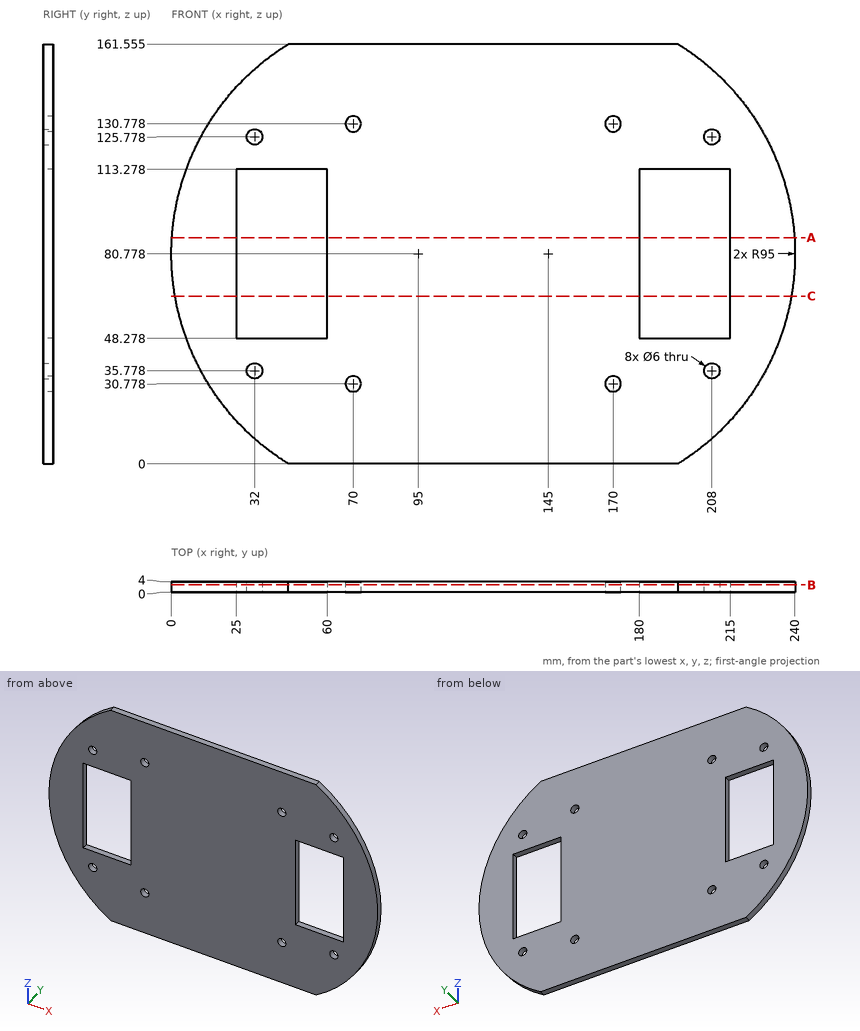
The drawing under review shows one solid part. Ordinate dimensions are in mm from its lowest x, y, z. Round coordinates to 2 decimals unless told otherwise and drop trailing zeros. Order: outer loops, then holes, each group sorted by start corner. A loop starts at its lowest first (then second) coordinate and runs counter-clockwise, first axis right, second up. Notation, with made-up numbers: (67, 20.5) -> (76, 20.5) arc R6 cw to (76, 24.5) -> close; hole circle Ø10 at (-1.75, -15.75). An arc over 180 degrees is marked (long way). Use a Markdown table: item, result.
Q1. We need section C-C on z = 64.5. Write out the cut boundary in (x, y) (1 decimal).
Values:
| item | result |
|---|---|
| outline | (1.4, 0) -> (25, 0) -> (25, 4) -> (1.4, 4) -> close; (60, 0) -> (180, 0) -> (180, 4) -> (60, 4) -> close; (215, 0) -> (238.6, 0) -> (238.6, 4) -> (215, 4) -> close |
Q2. Clearance check with flat-ended pins moving along their axes: P1, Ø2, axis at x = 36.5, y = 2, coming from the +Z side; P2, Ø7, axis at x = 170, z = 130.78, coming from the +Y side; P3, Ø5, axis at x = 208, z = 125.78, coming from the +Y side; P4, Ø2, axis at x = 205.5, y = 2, coming from the +Z side (1 decimal). State where each tip first meets the part, or that it passes through.
Values:
| item | result |
|---|---|
| P1 | stops at z = 156.4 |
| P2 | stops at y = 4 |
| P3 | passes through |
| P4 | stops at z = 154.8 |
Q3. We need section A-A on z = 87. Write out the cut boundary in (x, y) (1 decimal).
Values:
| item | result |
|---|---|
| outline | (0.2, 0) -> (25, 0) -> (25, 4) -> (0.2, 4) -> close; (60, 0) -> (180, 0) -> (180, 4) -> (60, 4) -> close; (215, 0) -> (239.8, 0) -> (239.8, 4) -> (215, 4) -> close |
Q4. We need section B-B on y = 2.85. State how many separate pieces and enclosed holes the cut face has, then the cut area to 3 significant figures.
Values:
| item | result |
|---|---|
| separate pieces | 1 |
| enclosed holes | 10 |
| area | 29,700 mm^2 |
Q5. For line 1 (Z direction, x = 170, y = 2.95) (1 decimal); line 2 (X direction, y = 1.3, z = 80.5); line 3 (Z direction, x = 190.5, y = 2.35) (1 decimal), list the stretches that pass through material, from the lowest coordinate up.
Values:
| item | result |
|---|---|
| line 1 | z = 0 to 27.8, 33.8 to 127.8, 133.8 to 161.6 |
| line 2 | x = 0 to 25, 60 to 180, 215 to 240 |
| line 3 | z = 0 to 48.3, 113.3 to 161.6 |
